Design review of the part shown in the three views and the two pictorial views. Dimensions are in mm from the part's minimum x, y and z. A direction names the side the tool comes from. Round coordinates to 2 decimals unless told otherwise and drop trailing zeros. Order: outer loops, then holes, each group sorted by start corner. A loop starts at its lowest first (then second) coordinate and runs counter-clockwise, first axis right, second up.
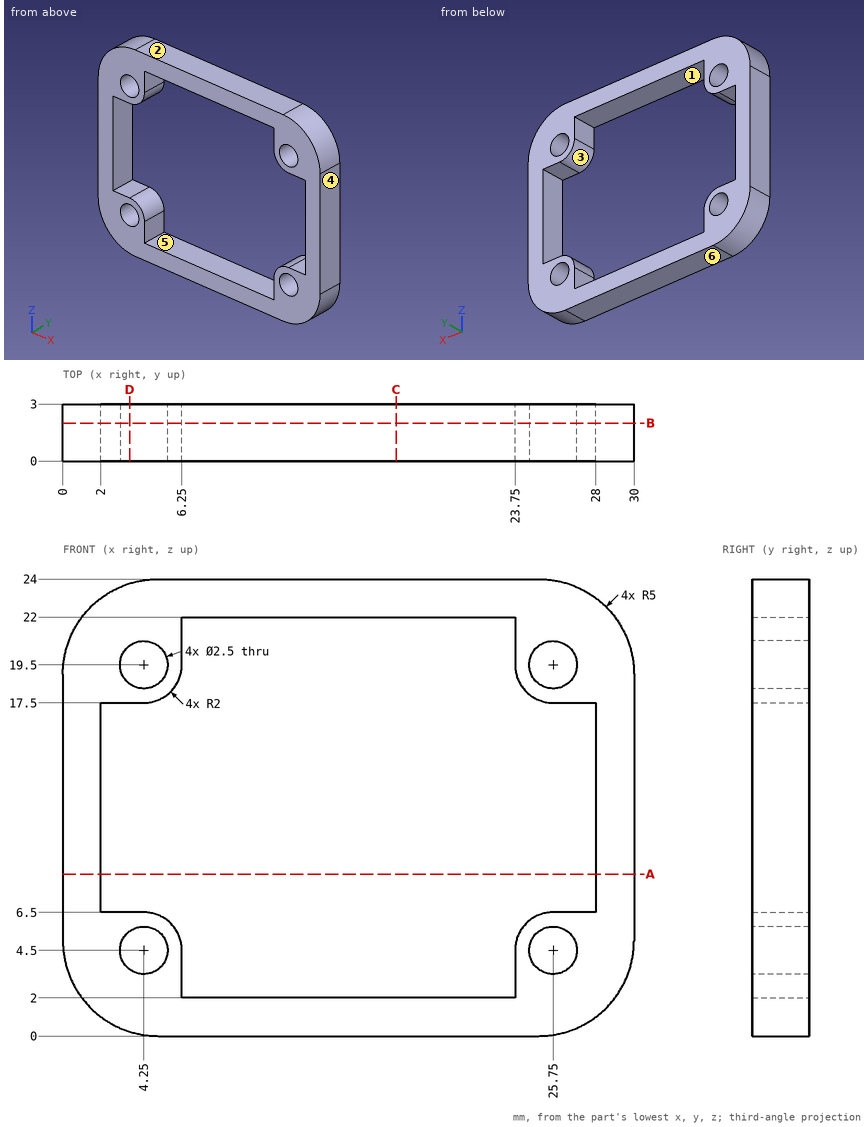
(1) Consider section D-D (x = 3.5). Write out the cut boundary in (y, z), and give its area (3 significant figures).
Data:
outline: (0, 0.23) - (3, 0.23) - (3, 3.5) - (0, 3.5) - close; (0, 5.5) - (3, 5.5) - (3, 6.5) - (0, 6.5) - close; (0, 17.5) - (3, 17.5) - (3, 18.5) - (0, 18.5) - close; (0, 20.5) - (3, 20.5) - (3, 23.77) - (0, 23.77) - close
area: 25.6 mm2
(2) Consider section C-C (x = 17.5). Write out the cut boundary in (y, z), and give its area (3 significant figures).
Data:
outline: (0, 0) - (3, 0) - (3, 2) - (0, 2) - close; (0, 22) - (3, 22) - (3, 24) - (0, 24) - close
area: 12.0 mm2
(3) Insertion check: pin 1 (1.1 mm diameter, centred on x = 3.5, y = 1.5, fed in from +Z); pin 2 (2 mm diameter, centred on x = 25.75, z = 4.5, fed in from -Y); pin 3 (0.8 mm diameter, centred on y = 2, z = 21.5, fed in from +X). Each pin has a flat end and moves straight along its axis. Give the tip position at first contact, or say it passes through.
Data:
pin 1: stops at z = 23.91
pin 2: passes through
pin 3: stops at x = 29.54
(4) For the marked faces 5 and 6, list the 3-axis set-ups (+Z, -Z, +X, -X, +Y, -Y) from which the entire face can be reached by the end or side of a thin tool; tool diameter is ignored.
Data:
face 5: +Y, -Y
face 6: -Z, +X, -X, +Y, -Y
(5) To check wall thickness, follow probe 1 along X at (y, z) = (1.75, 7.75); probe 2 along Z at (x, y) = (25.75, 2); probe 3 along X at (y, z) = (0.75, 4.5). State the ranges of each line that lie inside material, in increasing order.
Data:
probe 1: x = 0 to 2, 28 to 30
probe 2: z = 0.06 to 3.25, 5.75 to 6.5, 17.5 to 18.25, 20.75 to 23.94
probe 3: x = 0.03 to 3, 5.5 to 6.25, 23.75 to 24.5, 27 to 29.97
(6) Consider section A-A (z = 8.5). Write out the cut boundary in (x, y), and give its area (3 significant figures).
Data:
outline: (0, 0) - (2, 0) - (2, 3) - (0, 3) - close; (28, 0) - (30, 0) - (30, 3) - (28, 3) - close
area: 12.0 mm2
(7) Consider section B-B (y = 2). Write out the cut boundary in (x, z), and give its area (3 significant figures).
Data:
outline: (0, 5) arc R5 ccw to (5, 0) - (25, 0) arc R5 ccw to (30, 5) - (30, 19) arc R5 ccw to (25, 24) - (5, 24) arc R5 ccw to (0, 19) - close; hole (2, 6.5) - (4.25, 6.5) arc R2 cw to (6.25, 4.5) - (6.25, 2) - (23.75, 2) - (23.75, 4.5) arc R2 cw to (25.75, 6.5) - (28, 6.5) - (28, 17.5) - (25.75, 17.5) arc R2 cw to (23.75, 19.5) - (23.75, 22) - (6.25, 22) - (6.25, 19.5) arc R2 cw to (4.25, 17.5) - (2, 17.5) - close; hole circle Ø2.5 at (4.25, 4.5); hole circle Ø2.5 at (4.25, 19.5); hole circle Ø2.5 at (25.75, 4.5); hole circle Ø2.5 at (25.75, 19.5)
area: 232 mm2
(8) Draft analysis for pull direction Z (two halves, no side actions). For the marked faces 1, 2, 3 and 4, state which applies: pulls with the +Z half, pulls with the -Z half, needs draft (parallel to the pull), parting line crosses it, or undercut.
Data:
face 1: undercut
face 2: pulls with the +Z half
face 3: undercut
face 4: needs draft
